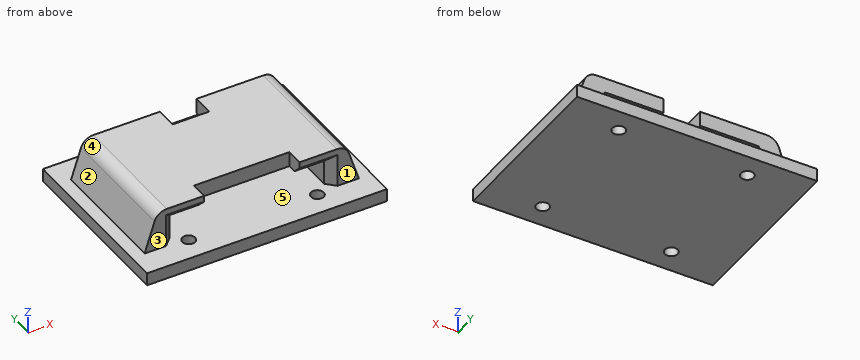
from build123d import *

# Parameters (mm, degrees)
F1_DEPTH  = 3.5
F2_W      = 29
F2_H      = 9.2
F3_DEPTH  = 4
F4_W      = 29
F4_H      = 9.2
F5_DEPTH  = 4
F6_SIZE   = 2
F7_W      = 4
F7_H      = 15
F8_DEPTH  = 3
F9_SIZE   = 2
F11_DEPTH = 29
F12_R     = 3
F13_W     = 56
F13_H     = 41
F14_DEPTH = 3
F15_R     = 1.5
F16_DEPTH = 3


with BuildPart() as f1:
    # F0 (on Top) → F1 (new body)
    with BuildSketch(Plane.XY):
        Polygon((-4.25, 12.1511180716), (-18, 12.1511180716), (-18, -16.8488819284), (-11.125, -16.8488819284), (-11.125, -12.8488819284), (11.125, -12.8488819284), (11.125, -16.8488819284), (18, -16.8488819284), (18, 12.1511180716), (4.25, 12.1511180716), (4.25, 7.1511180716), (-4.25, 7.1511180716), align=None)
    extrude(amount=F1_DEPTH)

    # F2 (on face) → F3 (join)
    with BuildSketch(Plane(origin=(-18, 0, 0), x_dir=(0, -1, 0), z_dir=(-1, 0, 0))):
        with Locations((2.3488819284, -1.1)):
            Rectangle(F2_W, F2_H)
    extrude(amount=F3_DEPTH)

    # F4 (on face) → F5 (join)
    with BuildSketch(Plane.YZ.offset(18)):
        with Locations((-2.3488819284, -1.1)):
            Rectangle(F4_W, F4_H)
    extrude(amount=F5_DEPTH)

    # F6
    f6_edges = [f1.edges().sort_by_distance(p)[0] for p in [
        (-14.5625, -16.848882, 0),
        (14.5625, -16.848882, 0),
    ]]
    chamfer(f6_edges, length=F6_SIZE)

    # F7 (on face) → F8 (join)
    with BuildSketch(Plane(origin=(0, 0, -5.7), x_dir=(1, 0, 0), z_dir=(0, 0, -1))):
        with Locations((20, 2.3488819284)):
            Rectangle(F7_W, F7_H)
        with Locations((-20, 2.3488819284)):
            Rectangle(F7_W, F7_H)
    extrude(amount=F8_DEPTH)

    # F9
    f9_edges = [f1.edges().sort_by_distance(p)[0] for p in [
        (18, -16.848882, -1.85),
        (-18, -16.848882, -1.85),
    ]]
    chamfer(f9_edges, length=F9_SIZE)

    # F10 (on face) → F11 (join, through all)
    with BuildSketch(Plane(origin=(0, 12.1511180716, 0), x_dir=(-1, 0, 0), z_dir=(0, 1, 0))):
        Polygon((25, -5.7), (22, 3.5), (22, -5.7), align=None)
        Polygon((-22, -5.7), (-22, 3.5), (-25, -5.7), align=None)
    extrude(amount=-F11_DEPTH)

    # F12
    f12_edges = [f1.edges().sort_by_distance(p)[0] for p in [
        (-22, -2.348882, 3.5),
        (22, -2.348882, 3.5),
    ]]
    fillet(f12_edges, radius=F12_R)

    # F13 (on face) → F14 (join, through all)
    with BuildSketch(Plane(origin=(0, 0, -5.7), x_dir=(1, 0, 0), z_dir=(0, 0, -1))):
        with Locations((0, 2.3488819284)):
            Rectangle(F13_W, F13_H)
    extrude(amount=F14_DEPTH)

    # F15 (on face) → F16 (cut, through all)
    with BuildSketch(Plane(origin=(0, 0, -8.7), x_dir=(1, 0, 0), z_dir=(0, 0, -1))):
        with Locations((-15, 17.3488819284)):
            Circle(F15_R)
        with Locations((15, 17.3488819284)):
            Circle(F15_R)
        with Locations((15, -12.6511180716)):
            Circle(F15_R)
        with Locations((-15, -12.6511180716)):
            Circle(F15_R)
    extrude(amount=-F16_DEPTH, mode=Mode.SUBTRACT)


solid = f1.part
Source: CAD feature listing. Evaluate the final solid. Frame: model axes, mm. Face numbers are marked on the shaded views. A direction names the side the tool comes from. Coordinates: 2 decimals unless noted, no trailing zeros. Loops run counter-clockwise (first coordinate to the right, second up) from the corner with the lowest first, then second, coordinate; pieces in that order, holes last. Notation, with made-up numbers: (15.5, 48.5) -> (35.5, 48.5) arc R27 cw to (35.5, 72.5) -> close; hole circle Ø11 at (-38.5, 74.25). An arc over 180 degrees is marked (long way). Answer in a Markdown table with one row per item. Add a question column.
Q1. Reachability of the marked faces 1 and 2 from +Z, -Z, +X, -X, +Y, -Y: full face, straight path, thin tool, end or side. Return the list, or none.
Q2. Ray query, line 1 along Y through (x, z) = (-15, -7.6); line 2 along Z through (x, y) = (13.5, 11); line 3 along Y through (x, z) = (-18, 2.5). Return the intervals inside material, ascending.
Q3. Pull-direction query (Z, two-part tool) for the marked faces 3, 4 and 5; classes: pulls with the +Z half, pulls with the -Z half, needs draft (parallel to the pull), parting line crosses it, or undercut.
Q4. Section B-B on x = 8. Return the cut outline in (y, z).
Q5. Section D-D on x = -15. Return the cut outline in (y, z).
Q6. Contact query for flat-ended pins moving along their axis: pin 1 Ø4 at (x, z) = (-18.5, -2.5) entering from -Y; pin 2 Ø1.5 at (y, z) = (-7, -3.5) entering from -X; pin 3 Ø1 at (y, z) = (9.5, 1) entering from -X. Output: stop coordinate, or through.
Q7. Section C-C on z = -3. Return the cut outline in (x, y).
Q8. Section A-A on y = -0.5. Return the cut outline in (x, z).
Computed values:
| question | item | result |
|---|---|---|
| 1 | face 1 | +Z, +X, -X, -Y |
| 1 | face 2 | +Z, -X, +Y, -Y |
| 2 | line 1 | y = -22.85 to -18.85, -15.85 to 11.15, 14.15 to 18.15 |
| 2 | line 2 | z = -8.7 to -5.7, 0 to 3.5 |
| 2 | line 3 | y = -16.85 to 12.15 |
| 3 | face 3 | needs draft |
| 3 | face 4 | pulls with the +Z half |
| 3 | face 5 | undercut |
| 4 | outline | (-22.85, -8.7) -> (18.15, -8.7) -> (18.15, -5.7) -> (-22.85, -5.7) -> close; (-12.85, 0) -> (12.15, 0) -> (12.15, 3.5) -> (-12.85, 3.5) -> close |
| 5 | outline | (-22.85, -8.7) -> (-18.85, -8.7) -> (-18.85, -5.7) -> (-22.85, -5.7) -> close; (-16.85, 2) -> (-14.85, 0) -> (12.15, 0) -> (12.15, 3.5) -> (-16.85, 3.5) -> close; (-15.85, -8.7) -> (11.15, -8.7) -> (11.15, -5.7) -> (-15.85, -5.7) -> close; (14.15, -8.7) -> (18.15, -8.7) -> (18.15, -5.7) -> (14.15, -5.7) -> close |
| 6 | pin 1 | stops at y = -16.85 |
| 6 | pin 2 | stops at x = -24.53 |
| 6 | pin 3 | stops at x = -22.98 |
| 7 | outline | (-24.12, -16.85) -> (-20, -16.85) -> (-18, -14.85) -> (-18, 12.15) -> (-24.12, 12.15) -> close; (18, -14.85) -> (20, -16.85) -> (24.12, -16.85) -> (24.12, 12.15) -> (18, 12.15) -> close |
| 8 | outline | (-28, -8.7) -> (28, -8.7) -> (28, -5.7) -> (25, -5.7) -> (22.67, 1.43) arc R3 ccw to (19.82, 3.5) -> (-19.82, 3.5) arc R3 ccw to (-22.67, 1.43) -> (-25, -5.7) -> (-28, -5.7) -> close; hole (-18, -5.7) -> (18, -5.7) -> (18, 0) -> (-18, 0) -> close |
